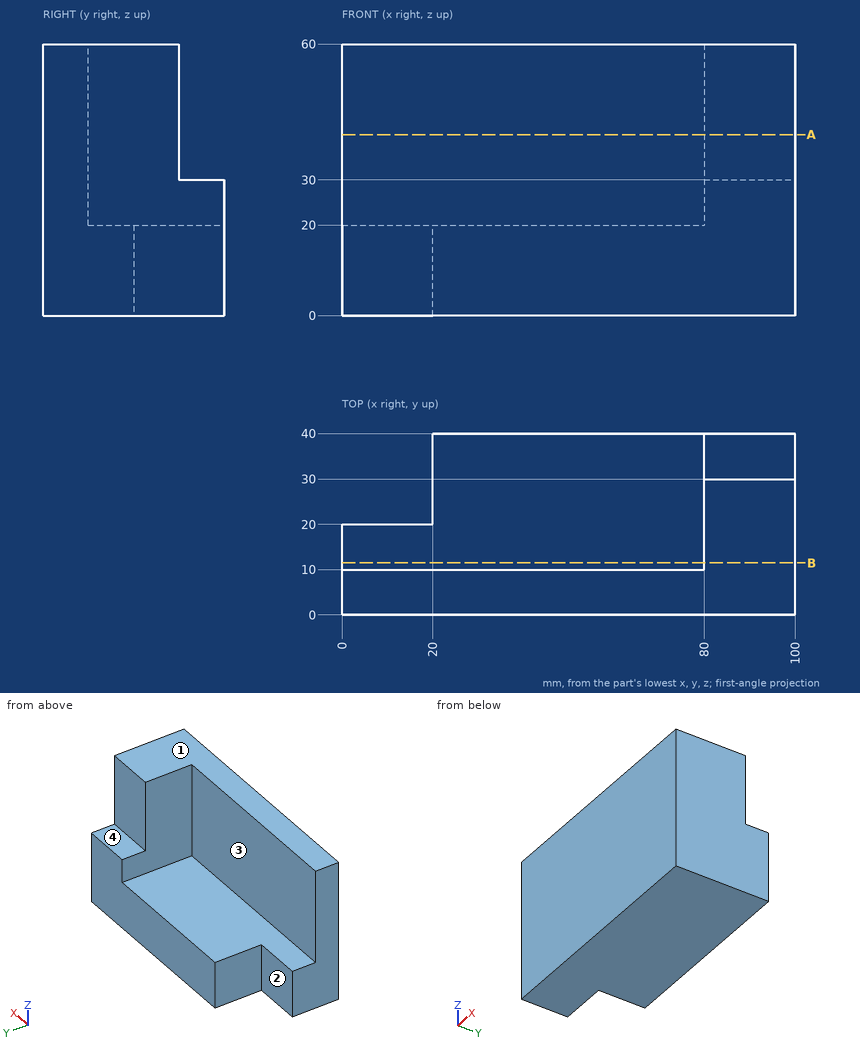
Source: three-view drawing plus pictorial views. Frame: mm from the lowest corner of the part. A direction names the side the tool comes from. Coordinates: 2 decimals unless noted, no trailing zeros. Loops run counter-clockwise (first coordinate to the right, second up) from the corner with the lowest first, then second, coordinate; pieces in that order, holes last. Notation, with made-up numbers: (37.5, -7.75) -> (82.5, -7.75) arc R5 ccw to (82.5, -0.75) -> close; hole circle Ø4 at (-21, 26.25). An arc over 180 degrees is marked (long way). Answer in a Markdown table with one row per item. Add a question column.
Q1. Ray query, line 1 along Y through (x, z) = (57, 43); line 2 along Z through (x, y) = (83, 36); line 3 along X through (y, z) = (15, 31). Return the intervals inside material, ascending.
Q2. Reachability of the marked faces 1, 2, 3 and 4 from +Z, -Z, +X, -X, +Y, -Y: full face, straight path, thin tool, end or side. Return the list, or none.
Q3. Section A-A on z = 40. Return the cut outline in (x, y), and give its area (3 significant figures).
Q4. Contact query for flat-ended pins moving along their axis: pin 1 Ø4 at (x, z) = (71, 24) entering from +Y; pin 2 Ø15 at (x, y) = (32.5, 31) entering from +Z; pin 3 Ø10 at (y, z) = (30.5, 7.5) entering from -X. Output: stop coordinate, or through.
Q5. Section B-B on y = 11.5. Return the cut outline in (x, z).
Computed values:
| question | item | result |
|---|---|---|
| 1 | line 1 | y = 0 to 10 |
| 1 | line 2 | z = 0 to 30 |
| 1 | line 3 | x = 80 to 100 |
| 2 | face 1 | +Z, +X, -X, +Y, -Y |
| 2 | face 2 | +Z, -Z, -X, +Y |
| 2 | face 3 | +Z, -X, +Y |
| 2 | face 4 | +Z, +X, -X, +Y |
| 3 | outline | (0, 0) -> (100, 0) -> (100, 30) -> (80, 30) -> (80, 10) -> (0, 10) -> close |
| 3 | area | 1,400 mm^2 |
| 4 | pin 1 | stops at y = 10 |
| 4 | pin 2 | stops at z = 20 |
| 4 | pin 3 | stops at x = 20 |
| 5 | outline | (0, 0) -> (100, 0) -> (100, 60) -> (80, 60) -> (80, 20) -> (0, 20) -> close |
